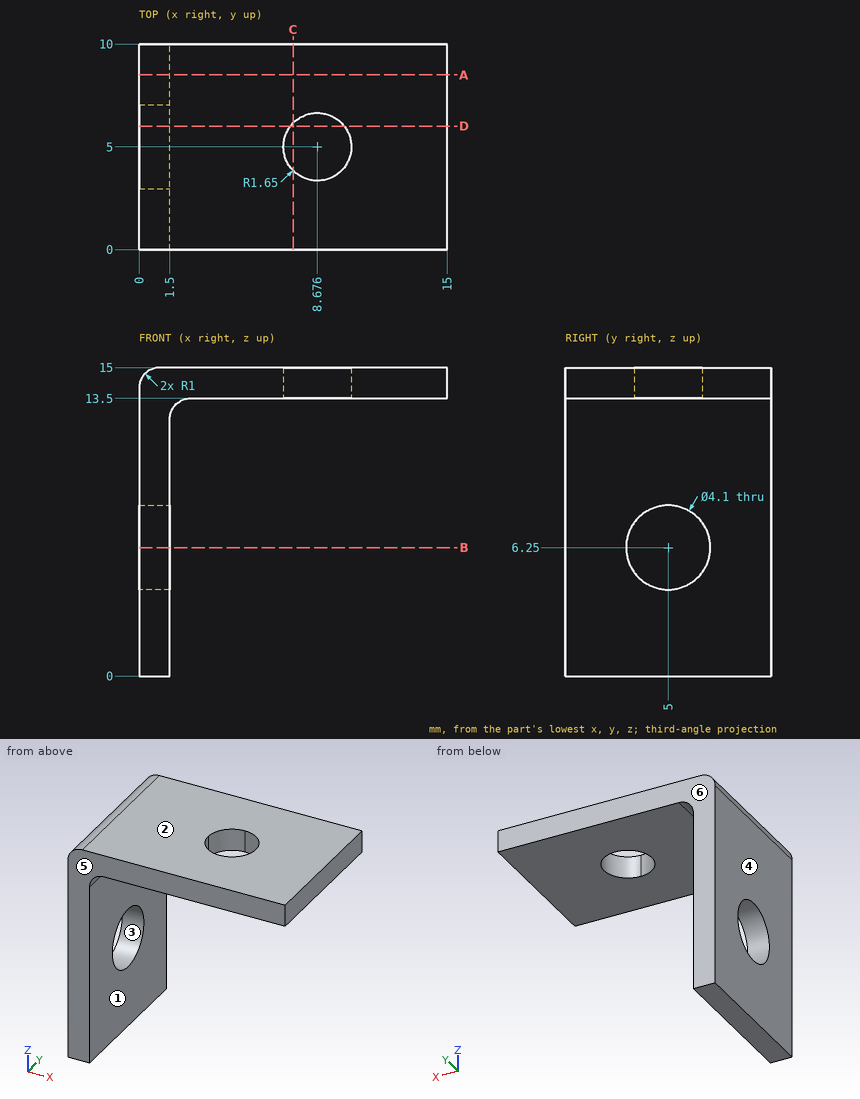
Study the drawing (mm; zero at the part's minimum x, y, z) and answer. A direction names the side the tool comes from. Give positions to 0.01 mm unless a question says otherwise; leave off trailing zeros. Loops run counter-clockwise (first coordinate to the right, second up) from the corner with the lowest first, then second, coordinate; pieces in that order, holes last. Notation, with made-up numbers: (41.5, -33) - (55.5, -33) arc R11 ccw to (55.5, -22) - close; hole circle Ø11 at (26, -29.5). An arc over 180 degrees is marked (long way). Return JSON: item names as keys, results as strings. Group by question number.
1. Straight lines are drawn through the part: line 1 (Y direction, x = 0.6, z = 6.25); line 2 (X direction, y = 6.5, z = 10); line 3 (Z direction, x = 13.5, y = 6). For each, find the intervals that lie inside material, in ascending order. Write a range as [from, to].
2. Find section C-C (x = 7.5). Write down the section's boundary in (y, z), then the cut area to 3 significant figures.
3. Find section D-D (y = 6). Write down the section's boundary in (x, z).
4. Determine the mould class of the marked faces 3, 4, 5 and 6 for opening direction Y: pulls with the +Y half, pulls with the -Y half, needs draft (parallel to the pull), parting line crosses it, or undercut.
5. Find section A-A (y = 8.5). Write down the section's boundary in (x, z).
6. Find section B-B (z = 6.25). Write down the section's boundary in (x, y).
7. Given pin 1 Ø2 at (x, y) = (12.5, 4) entering from -Z; pin 2 Ø1.5 at (y, z) = (1.5, 2) entering from +X, each flat-ended and moving along its own axis, determine where each tip first touches the part or whether it passes through.
8. Which of the six approach directions +Z, -Z, +X, -X, +Y, -Y give full straight-line access (tool end or side, diameter ignored) to the marked faces 1 and 2?
Verdict:
{
 "1": {"line 1": "y = [0, 2.95], [7.05, 10]", "line 2": "x = [0, 1.5]", "line 3": "z = [13.5, 15]"},
 "2": {"outline": "(0, 13.5) - (3.84, 13.5) - (3.84, 15) - (0, 15) - close; (6.16, 13.5) - (10, 13.5) - (10, 15) - (6.16, 15) - close", "area": "11.5 mm^2"},
 "3": {"outline": "(0, 0) - (1.5, 0) - (1.5, 4.46) - (0, 4.46) - close; (0, 8.04) - (1.5, 8.04) - (1.5, 12.5) arc R1 cw to (2.5, 13.5) - (7.36, 13.5) - (7.36, 15) - (1, 15) arc R1 ccw to (0, 14) - close; (9.99, 13.5) - (15, 13.5) - (15, 15) - (9.99, 15) - close"},
 "4": {"face 3": "undercut", "face 4": "needs draft", "face 5": "pulls with the -Y half", "face 6": "pulls with the +Y half"},
 "5": {"outline": "(0, 0) - (1.5, 0) - (1.5, 12.5) arc R1 cw to (2.5, 13.5) - (15, 13.5) - (15, 15) - (1, 15) arc R1 ccw to (0, 14) - close"},
 "6": {"outline": "(0, 0) - (1.5, 0) - (1.5, 2.95) - (0, 2.95) - close; (0, 7.05) - (1.5, 7.05) - (1.5, 10) - (0, 10) - close"},
 "7": {"pin 1": "stops at z = 13.5", "pin 2": "stops at x = 1.5"},
 "8": {"face 1": "-Z, +X, +Y, -Y", "face 2": "+Z, +X, -X, +Y, -Y"}
}
